Read the model definition and answer for the solid it produces. Units are mm, in the model's axes. Face numbers are marked on the shaded views. A direction names the side the tool comes from. Coordinates: 2 decimals unless noted, no trailing zeros. Order: outer loops, then holes, each group sorted by start corner. A loop starts at its lowest first (then second) coordinate and runs counter-clockwise, first axis right, second up. Notation, with made-up numbers: (26.25, -39.75) -> (64.25, -39.75) arc R25 cw to (64.25, -2.75) -> close; hole circle Ø3 at (60.5, 50.25). An arc over 180 degrees is marked (long way). Use CSV: the item, a comma, the result in double quotes.
```python
from build123d import *

# Parameters (mm, degrees)
EXTRUDE_1_DEPTH = 40
SKETCH_3_W      = 15
SKETCH_3_H      = 40
EXTRUDE_3_DEPTH = 10


with BuildPart() as part:
    # 草图1 → 凸台-拉伸1 (new body)
    with BuildSketch(Plane.XY):
        with BuildLine():
            Line((-125, 0), (-140, 0))
            ThreePointArc((-140, 0), (0, 140), (140, 0))
            Line((140, 0), (125, 0))
            ThreePointArc((125, 0), (0, 125), (-125, 0))
        make_face()
    extrude(amount=EXTRUDE_1_DEPTH)

    # 草图3 → 凸台-拉伸3 (add)
    with BuildSketch(Plane.XZ):
        with Locations((132.5, 20)):
            Rectangle(SKETCH_3_W, SKETCH_3_H)
    extrude(amount=EXTRUDE_3_DEPTH)


solid = part.part
```
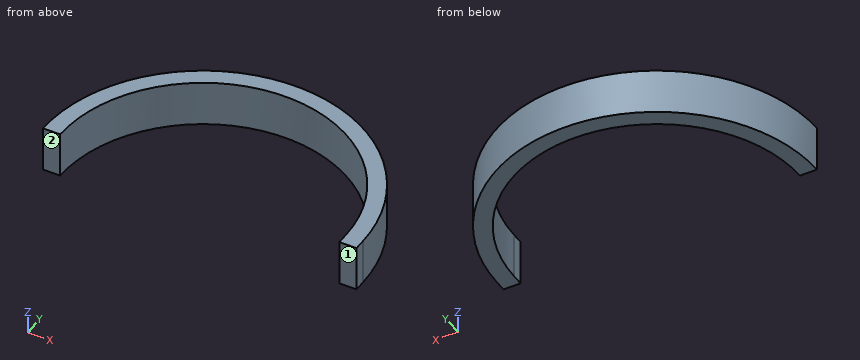
Item 1: Find section A-A, the plane y = 40. Give the vertices of the cut face in (x, z), then the cut area to 3 significant figures.
Return value:
outline,"(-134.16, 0) -> (-118.43, 0) -> (-118.43, 40) -> (-134.16, 40) -> close; (118.43, 0) -> (134.16, 0) -> (134.16, 40) -> (118.43, 40) -> close"
area,"1,260 mm^2"
Item 2: A tool of negligible diameter and unlimited length cuts with its end or side. For the marked faces 1 and 2, from which of +Z, -Z, +X, -X, +Y, -Y can it reach the whole face along a straight path? Write none if from no direction.
Return value:
face 1,"+Z, -Z, +X, -X, -Y"
face 2,"+Z, -Z, -X, -Y"
Item 3: Find section D-D, the plane x = 0. Give the vertices of the cut face in (y, z), then the cut area to 3 significant figures.
Return value:
outline,"(125, 0) -> (140, 0) -> (140, 40) -> (125, 40) -> close"
area,"600 mm^2"
Item 4: Each of these flat-tipped pins is pushed along its axis until it touches: P1, Ø16.5, axis at x = -136, z = 28, coming from the -Y side; P2, Ø1.5, axis at x = 97, z = 35, coming from the -Y side; P3, Ø1, axis at x = 26.5, z = 8, coming from the -Y side. Where does it stop, or does it pass through?
Return value:
P1,"stops at y = 0"
P2,"stops at y = 77.91"
P3,"stops at y = 122.05"
Item 5: Straight lines are drawn through the part: line 1 along X through (y, z) = (3.5, 6.5); line 2 along X through (y, z) = (57, 8); line 3 along Y through (x, z) = (-3, 31). For each, find the intervals that lie inside material, in ascending order.
Return value:
line 1,"x = -139.96 to -124.95, 124.95 to 139.96"
line 2,"x = -127.87 to -111.25, 111.25 to 127.87"
line 3,"y = 124.96 to 139.97"
Item 6: Find section B-B, the plane z = 5. Give the vertices of the cut face in (x, y).
Return value:
outline,"(-140, 0) -> (-125, 0) arc R125 cw to (125, 0) -> (125, -10) -> (140, -10) -> (140, 0) arc R140 ccw to start"
Item 7: Find section C-C, the plane y = 99. Give the vertices of the cut face in (x, z).
Return value:
outline,"(-98.99, 0) -> (-76.32, 0) -> (-76.32, 40) -> (-98.99, 40) -> close; (76.32, 0) -> (98.99, 0) -> (98.99, 40) -> (76.32, 40) -> close"
